from build123d import *
from build123d.topology import SkipClean

# Parameters (mm, degrees)
SKETCH_1_W          = 130.33985981
SKETCH_1_H          = 92
SKETCH_1_R          = 2
SKETCH_1_R_2        = 1.785582523
SKETCH_1_R_3        = 1.95
EXTRUDE_1_DEPTH     = 1
EXTRUDE_START       = -24
SKETCH_2_R          = 2
EXTRUDE_2_DEPTH     = 5
EXTRUDE_START_2     = 6
SKETCH_3_W          = 40
SKETCH_3_H          = 30
SKETCH_3_R          = 1.95
EXTRUDE_3_DEPTH     = 6
CUT_EXTRUDE_START   = 4
SKETCH_5_R          = 1.95
CUT_EXTRUDE_3_DEPTH = 6


with BuildPart() as part:
    # 草图1 → 凸台-拉伸1 (new, symmetric)
    with BuildSketch(Plane.XY):
        with Locations((65.169929905, 43)):
            Rectangle(SKETCH_1_W, SKETCH_1_H)
        with Locations((124.33985981, 10)):
            Circle(SKETCH_1_R, mode=Mode.SUBTRACT)
        with Locations((124.33985981, 76)):
            Circle(SKETCH_1_R, mode=Mode.SUBTRACT)
        with Locations((7, 3)):
            Circle(SKETCH_1_R, mode=Mode.SUBTRACT)
        with Locations((113, 3)):
            Circle(SKETCH_1_R_2, mode=Mode.SUBTRACT)
        with Locations((7, 83)):
            Circle(SKETCH_1_R, mode=Mode.SUBTRACT)
        with Locations((113, 83)):
            Circle(SKETCH_1_R, mode=Mode.SUBTRACT)
        with Locations((65.169929905, 50)):
            Circle(SKETCH_1_R_3, mode=Mode.SUBTRACT)
    extrude(amount=EXTRUDE_1_DEPTH, both=True)

    # 草图2 → 凸台-拉伸2 (add)
    with BuildSketch(Plane.XZ.offset(3).offset(EXTRUDE_START)):
        Polygon((62.24, 49.07), (72.24, 49.07), (87.24, 1), (62.24, 1), align=None)
        with Locations(Location((67.24, 44.07, 0), (0, 0, 270))):
            Circle(SKETCH_2_R, mode=Mode.SUBTRACT)
    extrude(amount=-EXTRUDE_2_DEPTH)

    # 草图3 → 凸台-拉伸3 (add)
    with SkipClean():  # the faces are left unmerged after this step: merging them gives an invalid solid
        with BuildSketch(Plane(origin=(0, 0, -1), x_dir=(-1, 0, 0), z_dir=(0, 0, -1)).offset(EXTRUDE_START_2)):
            with Locations((-65.169929905, 50)):
                Rectangle(SKETCH_3_W, SKETCH_3_H)
            with Locations((-79.836596572, 61)):
                Circle(SKETCH_3_R, mode=Mode.SUBTRACT)
            with Locations((-50.503263238, 61)):
                Circle(SKETCH_3_R, mode=Mode.SUBTRACT)
            with Locations((-50.503263238, 39)):
                Circle(SKETCH_3_R, mode=Mode.SUBTRACT)
            with Locations((-79.836596572, 39)):
                Circle(SKETCH_3_R, mode=Mode.SUBTRACT)
            with Locations((-65.169929905, 50)):
                Circle(SKETCH_3_R, mode=Mode.SUBTRACT)
        extrude(amount=-EXTRUDE_3_DEPTH)

    # 草图5 → 切除-拉伸3 (cut)
    with SkipClean():  # the faces are left unmerged after this step: merging them gives an invalid solid
        with BuildSketch(Plane(origin=(0, 0, -1), x_dir=(-1, 0, 0), z_dir=(0, 0, -1)).offset(CUT_EXTRUDE_START)):
            with Locations((-50.503263238, 39)):
                Circle(SKETCH_5_R)
            with Locations((-79.836596572, 39)):
                Circle(SKETCH_5_R)
            with Locations((-79.836596572, 61)):
                Circle(SKETCH_5_R)
            with Locations((-50.503263238, 61)):
                Circle(SKETCH_5_R)
        extrude(amount=-CUT_EXTRUDE_3_DEPTH, mode=Mode.SUBTRACT)


solid = part.part
Part model, mm, in its own coordinate system. A direction names the side the tool comes from. Round coordinates to 2 decimals unless told otherwise and drop trailing zeros. Write each loop counter-clockwise with the first axis right and the second up, starting at its lowest first coordinate (ties: lowest second). Pieces come first, ordered by that corner, then holes. Notation, with made-up numbers: M -11,81.5 L 15,81.5 A26 ccw 15,114.5 Z; hole C 45,25 d4. An arc over 180 degrees is marked long. Return JSON: item names as keys, results as strings. Group by question number.
(1) Saw through at D-D on z = 44.07. Write the cut outline in (x, y).
(2) Saw through at B-B on x = 113. Write the cut outline in (y, z), then the cut area to 3 significant figures.
(3) Saw through at A-A on y = 39. Write the cut outline in (x, z).
(4) Saw through at C-C on y = 22.5. Write the cut outline in (x, z), then the cut area to 3 significant figures.
(5) Which spindle directions (+Z, -Z, +X, -X, +Y, -Y) get a long thin tool onto all of the face, cutting with end or side? Do faces 1 (the face through (72, 21, 20)), 2 (the face through (85.17, 50, -4)), 3 (the face through (65, 65, -4)). Say none if no direction does.
(6) Drill centre lines: probe 1 along Y at (x, z) = (50.5, -4); probe 2 along Y at (x, z) = (7, -0.6); probe 3 along Z at (x, y) = (113, 72). Where is each one in solid material? Low to high.
(7) Two-plate mould, pull along X, no slides. Class faces 4 (the face through (79.635, 23.465, 25.371)), 5 (the face through (64, 44, 1)), 6 (the face through (5.4, 1.8, 0)): +X half, -X half, draft (parallel to the pull), parting line (faces both ways), or undercut.
(8) Pin check, flat tips, straight feed: pin 1 Ø4.5 at (x, y) = (50.5, 61) entering from +Z; pin 2 Ø8 at (x, y) = (25, 42) entering from -Z; pin 3 Ø1.8 at (x, z) = (66.5, -2.5) entering from +Y; pin 4 Ø2.5 at (x, y) = (79.84, 61) entering from +Z. Stop position of each tip, or through.
Returned:
{
 "1": {"outline": "M 62.24,21 L 65.24,21 L 65.24,26 L 62.24,26 Z; M 69.24,21 L 73.8,21 L 73.8,26 L 69.24,26 Z"},
 "2": {"outline": "M -3,-1 L 1.21,-1 L 1.21,1 L -3,1 Z; M 4.79,-1 L 81,-1 L 81,1 L 4.79,1 Z; M 85,-1 L 89,-1 L 89,1 L 85,1 Z", "area": "169 mm²"},
 "3": {"outline": "M 0,-1 L 45.17,-1 L 45.17,-7 L 48.55,-7 L 48.55,1 L 0,1 Z; M 52.45,-7 L 77.89,-7 L 77.89,1 L 52.45,1 Z; M 81.79,-7 L 85.17,-7 L 85.17,-1 L 130.34,-1 L 130.34,1 L 81.79,1 Z"},
 "4": {"outline": "M 0,-1 L 130.34,-1 L 130.34,1 L 87.24,1 L 72.24,49.07 L 62.24,49.07 L 62.24,1 L 0,1 Z; hole C 67.24,44.07 d4", "area": "1,090 mm²"},
 "5": {"face 1": "+Z, +X, -X, -Y", "face 2": "-Z, +X, +Y, -Y", "face 3": "-Z, +X, -X, +Y"},
 "6": {"probe 1": "35 to 37.05, 40.95 to 59.05, 62.95 to 65", "probe 2": "-3 to 1, 5 to 81, 85 to 89", "probe 3": "-1 to 1"},
 "7": {"face 4": "+X half", "face 5": "draft", "face 6": "undercut"},
 "8": {"pin 1": "z = 1", "pin 2": "z = -1", "pin 3": "y = 65", "pin 4": "through"}
}
